Part model, mm, in its own coordinate system. A direction names the side the tool comes from. Give positions to 0.01 mm unless a question says otherwise; leave off trailing zeros. Order: outer loops, then holes, each group sorted by start corner. A loop starts at its lowest first (then second) coordinate and runs counter-clockwise, first axis right, second up.
1. Mould opens along Z. For faces 4 (the cylindrical face through (39.856, 1.521, 3.279)), 5 (the flat face through (31, 12, 0)), 6 (the cylindrical face through (-56.39, 1.48, 16.58)) say: +Z half, -Z half, draft (parallel to the pull), parting line (faces both ways), or undercut.
2. Slice it at D-D on z = 10. List the corners of the cut face in (x, y).
3. Slice it at A-A on x = 45. List the corners of the cut face in (y, z), and give its area (3 significant figures).
4. Probe line 1 (X direction, y = 2.1, z = 0); line 2 (X direction, y = 24.5, z = -13.5); line 3 (X direction, y = 13, z = 14.5). List the from-to ranges inside material, lowest first.
5. Slice it at C-C on z = 0. Give the number of separate pieces and of enclosed holes in the cut face, and give its area (3 significant figures).
6. Drop flat-ended pins along their axis: pin 1 Ø3.5 at (x, z) = (28, 2.5) entering from -Y; pin 2 Ø1 at (y, z) = (23, -8) entering from -X; pin 3 Ø3.5 at (x, z) = (27, 1) entering from +Y. Give the stop position or say it passes through.
7. Which spindle directions (+Z, -Z, +X, -X, +Y, -Y) get a long thin tool onto all of the face, cutting with end or side? Do faces 1 (the flat face through (-31, 12, 0)), 2 (the flat face through (30, 4, 0)), 3 (the flat face through (49, 3, 5)). Say none if no direction does.
8. Slice it at B-B on y = 23.5. List the corners of the cut face in (x, z), and give its area (3 significant figures).
from build123d import *

# Parameters (mm, degrees)
EXTRUDE_THIN1_DEPTH = 20
SKETCH4_R           = 6.1
CUT_EXTRUDE3_DEPTH  = 69.767724988
FILLET1_R           = 12


with BuildPart() as part:
    # Sketch1 → Extrude-Thin1 (new, symmetric)
    with BuildSketch(Plane.XY):
        Polygon((-60, 0), (-30, 0), (-30, 9), (-25.5, 9), (-25.5, 18), (-21, 18), (-21, 27), (0, 27), (0, 30), (-24, 30), (-24, 21), (-28.5, 21), (-28.5, 12), (-33, 12), (-33, 3), (-60, 3), align=None)
    extrude_thin1 = extrude(amount=EXTRUDE_THIN1_DEPTH, both=True)

    # Mirror1: Extrude-Thin1 across plane
    add(extrude_thin1.mirror(Plane(origin=(0, 30, -20), x_dir=(0, 0, 1), z_dir=(-1, 0, 0))))

    # Sketch4 → Cut-Extrude3 (cut, through all)
    with BuildSketch(Plane(origin=(0, 3, 0), x_dir=(1, 0, 0), z_dir=(0, 1, 0))):
        with Locations(Location((-45, 0, 0), (0, 0, 270))):
            Circle(SKETCH4_R)
    cut_extrude3 = extrude(amount=-CUT_EXTRUDE3_DEPTH, mode=Mode.SUBTRACT)

    # Mirror3: Cut-Extrude3 across plane
    add(cut_extrude3.mirror(Plane(origin=(0, 0, 0), x_dir=(0, 0, 1), z_dir=(1, 0, 0))), mode=Mode.SUBTRACT)

    # Fillet1
    fillet1_edges = [part.edges().sort_by_distance(p)[0] for p in [
        (-60, 1.5, 20),
        (-60, 1.5, -20),
        (60, 1.5, -20),
        (60, 1.5, 20),
    ]]
    fillet(fillet1_edges, radius=FILLET1_R)


solid = part.part
Data:
1. face 4: undercut
1. face 5: draft
1. face 6: +Z half
2. outline: (-59.83, 0) - (-30, 0) - (-30, 9) - (-25.5, 9) - (-25.5, 18) - (-21, 18) - (-21, 27) - (21, 27) - (21, 18) - (25.5, 18) - (25.5, 9) - (30, 9) - (30, 0) - (59.83, 0) - (59.83, 3) - (33, 3) - (33, 12) - (28.5, 12) - (28.5, 21) - (24, 21) - (24, 30) - (-24, 30) - (-24, 21) - (-28.5, 21) - (-28.5, 12) - (-33, 12) - (-33, 3) - (-59.83, 3) - close
3. outline: (0, -20) - (3, -20) - (3, -6.1) - (0, -6.1) - close; (0, 6.1) - (3, 6.1) - (3, 20) - (0, 20) - close
3. area: 83.4 mm2
4. line 1: x = -60 to -51.1, -38.9 to -30, 30 to 38.9, 51.1 to 60
4. line 2: x = -24 to -21, 21 to 24
4. line 3: x = -28.5 to -25.5, 25.5 to 28.5
5. separate pieces: 3
5. enclosed holes: 0
5. area: 449 mm2
6. pin 1: stops at y = 9
6. pin 2: stops at x = -24
6. pin 3: stops at y = 21
7. face 1: +Z, -Z, -X, +Y
7. face 2: +Z, -Z, -Y
7. face 3: +Z, -Z, +X, +Y
8. outline: (-24, -20) - (-21, -20) - (-21, 20) - (-24, 20) - close; (21, -20) - (24, -20) - (24, 20) - (21, 20) - close
8. area: 240 mm2
